Here's how the part is built. I have some questions about the finished solid (model axes, mm). A direction names the side the tool comes from. Give positions to 0.01 mm unless a question says otherwise; leave off trailing zeros. Loops run counter-clockwise (first coordinate to the right, second up) from the corner with the lowest first, then second, coordinate; pieces in that order, holes last. Notation, with made-up numbers: (11.25, 12.25) - (68.25, 12.25) arc R25 cw to (68.25, 31.25) - close; hole circle Ø10 at (-31.75, -30). An arc over 180 degrees is marked (long way). Return JSON: item names as keys, results as strings. Group by question number.
(1) For P1, Ø2, axis at x = 36.5, z = 1, coming from the +Y side; P2, Ø1, axis at y = 39.5, z = 5, coming from the +X side; P3, Ø2, axis at y = 31.5, z = 1, coming from the +X side, each with a flat end and sliding along its axis, tell me the tip position at first contact or that it passes through.
(2) If we section it at C-C (x = 40.4): Please give me the cut outline in (y, z), then the cut area to 3 significant figures.
(3) If we section it at B-B (y = 48.8): Please give me the cut outline in (x, z), then the cut area to 3 significant figures.
(4) If we section it at D-D (z = 11.25): Please give me the cut outline in (x, y).
(5) If we section it at A-A (x = 30): Please give me the cut outline in (y, z).
(6) On a 3-axis mill with a long thin cutter (end or side, diameter ignored), from which of +Z, -Z, +X, -X, +Y, -Y can I reach the whole of each face in a straight line? I mean faces 1 (the flat face through (46.5, 30, 1)), 2 (the flat face through (23, 30, 0)), 3 (the cylindrical face through (54.8, 37.81, 8.41)). Say none if no direction works.
(7) If we mould it in two halves opening along Y, with no side actions, what happens to faces 4 (the cylindrical face through (6.99, 12.35, 7.4)), 5 (the flat face through (24, 30, 2)), 6 (the flat face through (26, 30, 1)), 7 (the flat face through (19, 54, 15))? For each: released by +Y, released by -Y, zero draft, split by the parting line, or undercut.
(8) I need wall thicknesses on probe 1 along X at (y, z) = (48.8, 1.5); probe 2 along Y at (x, z) = (22, 1.15); probe 3 along Y at (x, z) = (15, 11.25). Which ranges of each line are inside material? Lowest first, please. Write a range as [from, to].
```python
from build123d import *

# Parameters (mm, degrees)
PAD_DEPTH         = 10
CYLINDER002_R     = 2.5
CYLINDER002_DEPTH = 10
CYLINDER004_R     = 1.5
CYLINDER004_DEPTH = 10
CYLINDER003_R     = 1
CYLINDER003_DEPTH = 10
CYLINDER001_R     = 2.5
CYLINDER001_DEPTH = 10
CYLINDER005_R     = 26
CYLINDER005_DEPTH = 32
CYLINDER_R        = 29
CYLINDER_DEPTH    = 15


with BuildPart() as pad:
    # Sketch → Pad (new body)
    with BuildSketch(Plane.XY):
        with BuildLine():
            Line((27, 45), (45.5, 45))
            ThreePointArc((46.5, 44), (46.207107, 44.707107), (45.5, 45))
            Line((46.5, 44), (46.5, 16))
            ThreePointArc((45.5, 15), (46.207107, 15.292893), (46.5, 16))
            Line((45.5, 15), (27, 15))
            ThreePointArc((26, 16), (26.292893, 15.292893), (27, 15))
            Line((26, 16), (26, 44))
            ThreePointArc((27, 45), (26.292893, 44.707107), (26, 44))
        make_face()
    extrude(amount=PAD_DEPTH)


with BuildPart() as zylinder002:
    # Cylinder002 → Cylinder002 (new body)
    with BuildSketch(Plane(origin=(22, 50, -1), x_dir=(1, 0, 0), z_dir=(0, 0, 1))):
        Circle(CYLINDER002_R)
    extrude(amount=CYLINDER002_DEPTH)


with BuildPart() as zylinder004:
    # Cylinder004 → Cylinder004 (new body)
    with BuildSketch(Plane(origin=(8.08, 30.2, -1), x_dir=(1, 0, 0), z_dir=(0, 0, 1))):
        Circle(CYLINDER004_R)
    extrude(amount=CYLINDER004_DEPTH)


with BuildPart() as zylinder003:
    # Cylinder003 → Cylinder003 (new body)
    with BuildSketch(Plane(origin=(40.4, 48.8, -1), x_dir=(1, 0, 0), z_dir=(0, 0, 1))):
        Circle(CYLINDER003_R)
    extrude(amount=CYLINDER003_DEPTH)


with BuildPart() as fusion:
    # Cylinder001 → Cylinder001 (new body)
    with BuildSketch(Plane(origin=(22, 10, -1), x_dir=(1, 0, 0), z_dir=(0, 0, 1))):
        Circle(CYLINDER001_R)
    extrude(amount=CYLINDER001_DEPTH)

    # Fusion: union Pad, Zylinder002, Zylinder004, Zylinder003
    add(pad.part)
    add(zylinder002.part)
    add(zylinder004.part)
    add(zylinder003.part)


with BuildPart() as zylinder005:
    # Cylinder005 → Cylinder005 (new body)
    with BuildSketch(Plane(origin=(30, 30, 2), x_dir=(1, 0, 0), z_dir=(0, 0, 1))):
        Circle(CYLINDER005_R)
    extrude(amount=CYLINDER005_DEPTH)


with BuildPart() as cut001:
    # Cylinder → Cylinder (new body)
    with BuildSketch(Plane(origin=(30, 30, 0), x_dir=(1, 0, 0), z_dir=(0, 0, 1))):
        Circle(CYLINDER_R)
    extrude(amount=CYLINDER_DEPTH)

    # Cut: cut Zylinder005
    add(zylinder005.part, mode=Mode.SUBTRACT)

    # Cut001: cut Fusion
    add(fusion.part, mode=Mode.SUBTRACT)


solid = cut001.part
```
Values:
{
 "1": {"P1": "y = 58.47", "P2": "x = 57.57", "P3": "x = 59"},
 "2": {"outline": "(2.93, 0) - (15, 0) - (15, 2) - (6.17, 2) - (6.17, 15) - (2.93, 15) - close; (45, 0) - (47.8, 0) - (47.8, 2) - (45, 2) - close; (49.8, 0) - (57.07, 0) - (57.07, 15) - (53.83, 15) - (53.83, 2) - (49.8, 2) - close", "area": "129 mm2"},
 "3": {"outline": "(7.92, 0) - (19.81, 0) - (19.81, 2) - (12.04, 2) - (12.04, 15) - (7.92, 15) - close; (24.19, 0) - (39.4, 0) - (39.4, 2) - (24.19, 2) - close; (41.4, 0) - (52.08, 0) - (52.08, 15) - (47.96, 15) - (47.96, 2) - (41.4, 2) - close", "area": "183 mm2"},
 "4": {"outline": "circle Ø58 at (30, 30); hole circle Ø52 at (30, 30)"},
 "5": {"outline": "(1, 0) - (15, 0) - (15, 2) - (4, 2) - (4, 15) - (1, 15) - close; (45, 0) - (59, 0) - (59, 15) - (56, 15) - (56, 2) - (45, 2) - close"},
 "6": {"face 1": "+Z, -Z", "face 2": "-Z, +X, -X, +Y, -Y", "face 3": "+Z"},
 "7": {"face 4": "split by the parting line", "face 5": "undercut", "face 6": "undercut", "face 7": "zero draft"},
 "8": {"probe 1": "[7.92, 19.81], [24.19, 39.4], [41.4, 52.08]", "probe 2": "[2.13, 7.5], [12.5, 47.5], [52.5, 57.87]", "probe 3": "[5.18, 8.76], [51.24, 54.82]"}
}
